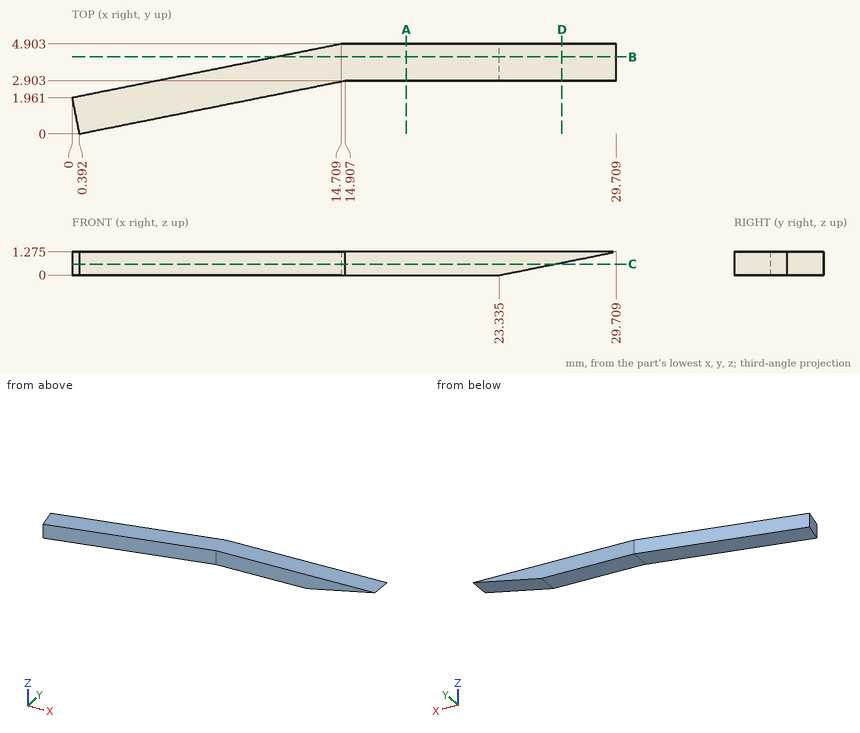
The figure shows three views and two pictorial views of one solid part (mm, origin at its lowest corner). Answer the questions. Coordinates: 2 decimals unless noted, no trailing zeros. Loops run counter-clockwise (first coordinate to the right, second up) from the corner with the lowest first, then second, coordinate; pieces in that order, holes last. Notation, with made-up numbers: M -33.5,14.25 L 24.5,14.25 A19 cw 24.5,20.25 Z; hole C 70,74.25 d2. An arc over 180 degrees is marked long. Use CSV: the item, a comma, the result in double quotes. Start each with the question number.
(1) Find section A-A, the plane x = 18.25. Give the vertices of the cut face in (y, z) (1 decimal).
(2) Find section C-C, the plane z = 0.6. Give the vertices of the cut face in (x, y) (1 decimal).
(3) Given pin 1 Ø0.6 at (x, z) = (20.5, 0.5) entering from -Y, flat-ended and moving along its own axis, determine where the tip first touches the part or whether it passes through.
(4) Find section D-D, the plane x = 26.75. Give the vertices of the cut face in (y, z) (1 decimal).
(5) Find section B-B, the plane y = 4.2. Give the vertices of the cut face in (x, z) (1 decimal).
(6) Consider line 1 (Y direction, x = 18.25, z = 0.85); line 2 (Y direction, x = 5.5, z = 0.8). Determine where each line is inside the solid, lowest interval first.
Recorded:
1,outline,"M 2.9,0 L 4.9,0 L 4.9,1.3 L 2.9,1.3 Z"
2,outline,"M 0,2 L 0.4,0 L 14.9,2.9 L 26.3,2.9 L 26.3,4.9 L 14.7,4.9 Z"
3,pin 1,"stops at y = 2.9"
4,outline,"M 2.9,0.7 L 4.9,0.7 L 4.9,1.3 L 2.9,1.3 Z"
5,outline,"M 11.2,0 L 23.3,0 L 29.7,1.3 L 11.2,1.3 Z"
6,line 1,"y = 2.9 to 4.9"
6,line 2,"y = 1.02 to 3.06"
